Job drawing, mm, ordinate dimensions from the low corner. One solid piece. Round coordinates to 2 decimals unless told otherwise and drop trailing zeros. Order: outer loops, then holes, each group sorted by start corner. A loop starts at its lowest first (then second) coordinate and runs counter-clockwise, first axis right, second up. Notation, with made-up numbers: (50.25, -22.75) -> (79.25, -22.75) arc R29 cw to (79.25, -2.75) -> close; hole circle Ø8 at (-29, 53.25). An arc over 180 degrees is marked (long way). Use CSV: the item, a comma, the result in double quotes.
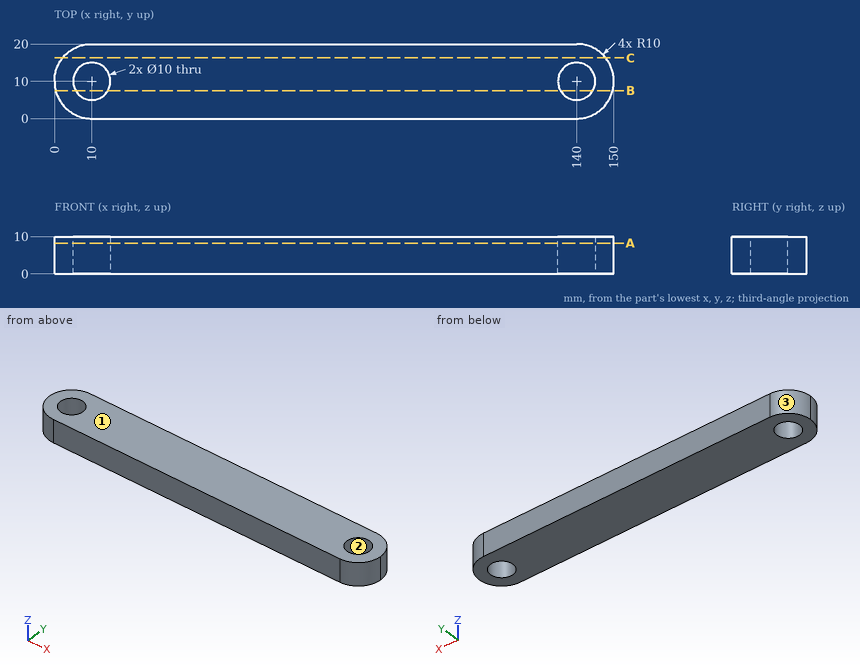
(1) Drop a flat-ended pin along its axis: P1, Ø5, axis at x = 54, y = 10.5, coming from the -Z side. Give the stop position or say it passes through.
Reply:
P1,"z = 0"
(2) Cut at C-C, the plane y = 16.25. Give the cut face in (x, z).
Reply:
outline,"(2.19, 0) -> (147.81, 0) -> (147.81, 10) -> (2.19, 10) -> close"
(3) Pull direction X, two halves, no side cores. Call the marked faces 1, 2 and 3: released by +X, released by -X, zero draft, split by the parting line, or undercut.
Reply:
face 1,"zero draft"
face 2,"undercut"
face 3,"released by -X"
(4) Probe probe 1 along Y at (x, z) = (10, 2); probe 2 along X at (y, z) = (13.5, 5.5); probe 3 along X at (y, z) = (7.75, 9) (1 decimal). List the from-to ranges inside material, lowest first. Write a range as [from, to].
Reply:
probe 1,"[0, 5], [15, 20]"
probe 2,"[0.63, 6.43], [13.57, 136.43], [143.57, 149.37]"
probe 3,"[0.3, 5.5], [14.5, 135.5], [144.5, 149.7]"
(5) Cut at B-B, the plane y = 7.5. Give the cut face in (x, z), then the cut area to 3 significant figures.
Reply:
outline,"(0.32, 0) -> (5.67, 0) -> (5.67, 10) -> (0.32, 10) -> close; (14.33, 0) -> (135.67, 0) -> (135.67, 10) -> (14.33, 10) -> close; (144.33, 0) -> (149.68, 0) -> (149.68, 10) -> (144.33, 10) -> close"
area,"1,320 mm2"
(6) Cut at A-A, the plane z = 8.25. State how many separate pieces and enclosed holes the cut face has, then the cut area to 3 significant figures.
Reply:
separate pieces,"1"
enclosed holes,"2"
area,"2,760 mm2"
